from build123d import *

# Parameters (mm, degrees)
SKETCH1_R               = 4.4
BOSS_EXTRUDE1_DEPTH     = 10
SKETCH1_2_R             = 4.4
BOSS_EXTRUDE2_DEPTH     = 2
SKETCH3_W               = 30
SKETCH3_H               = 12
BOSS_EXTRUDE4_DEPTH     = 7.2
CUT_EXTRUDE2_START      = -12.2
SKETCH2_R               = 1.65
CUT_EXTRUDE2_DEPTH      = 8
SKETCH5_W               = 30
SKETCH5_H               = 3
CUT_EXTRUDE3_DEPTH      = 23.756098084
CUT_EXTRUDE3_DEPTH_BACK = 2
SKETCH6_W               = 14
SKETCH6_H               = 3
CUT_EXTRUDE4_DEPTH      = 23.756098084
CUT_EXTRUDE4_DEPTH_BACK = 23.756098084


with BuildPart() as part:
    # Sketch1 → Boss-Extrude1 (new body)
    with BuildSketch(Plane.XY):
        with BuildLine():
            Line((-15, -5), (15, -5))
            ThreePointArc((15, -5), (10.104984149, -1.836764635), (6.785093744, 2.953388374))
            ThreePointArc((6.785093744, 2.953388374), (0, 7.4), (-6.785093744, 2.953388374))
            ThreePointArc((-6.785093744, 2.953388374), (-10.104984149, -1.836764635), (-15, -5))
        make_face()
        Circle(SKETCH1_R, mode=Mode.SUBTRACT)
    extrude(amount=BOSS_EXTRUDE1_DEPTH)

    # Sketch1<2> → Boss-Extrude2 (add)
    with BuildSketch(Plane.XY):
        with BuildLine():
            ThreePointArc((-6.785093744, 2.953388374), (0, 7.4), (6.785093744, 2.953388374))
            ThreePointArc((6.785093744, 2.953388374), (10.104984149, -1.836764635), (15, -5))
            Line((15, -5), (-15, -5))
            ThreePointArc((-15, -5), (-10.104984149, -1.836764635), (-6.785093744, 2.953388374))
        make_face()
        Circle(SKETCH1_2_R, mode=Mode.SUBTRACT)
        Circle(SKETCH1_2_R)
    extrude(amount=-BOSS_EXTRUDE2_DEPTH)

    # Sketch3 → Boss-Extrude4 (add)
    with BuildSketch(Plane.XZ.offset(5)):
        with Locations((0, 4)):
            Rectangle(SKETCH3_W, SKETCH3_H)
    extrude(amount=BOSS_EXTRUDE4_DEPTH)

    # Sketch2 → Cut-Extrude2 (cut)
    with BuildSketch(Plane(origin=(0, 0, 0), x_dir=(1, 0, 0), z_dir=(0, 1, 0)).offset(CUT_EXTRUDE2_START)):
        with Locations(Location((-11.5, -4, 0), (0, 0, 90))):
            Circle(SKETCH2_R)
        with Locations(Location((11.5, -4, 0), (0, 0, 90))):
            Circle(SKETCH2_R)
    extrude(amount=CUT_EXTRUDE2_DEPTH, mode=Mode.SUBTRACT)

    # Sketch5 → Cut-Extrude3 (cut, two sides)
    with BuildSketch(Plane(origin=(0, 0, -2), x_dir=(-1, 0, 0), z_dir=(0, 0, -1))) as cut_extrude3_sk:
        with Locations((0, -10.7)):
            Rectangle(SKETCH5_W, SKETCH5_H)
    extrude(amount=CUT_EXTRUDE3_DEPTH, mode=Mode.SUBTRACT)
    extrude(cut_extrude3_sk.sketch, amount=-CUT_EXTRUDE3_DEPTH_BACK, mode=Mode.SUBTRACT)

    # Sketch6 → Cut-Extrude4 (cut, two sides)
    with BuildSketch(Plane.XY.offset(10)) as cut_extrude4_sk:
        with Locations((0, -10.7)):
            Rectangle(SKETCH6_W, SKETCH6_H)
    extrude(amount=CUT_EXTRUDE4_DEPTH, mode=Mode.SUBTRACT)
    extrude(cut_extrude4_sk.sketch, amount=-CUT_EXTRUDE4_DEPTH_BACK, mode=Mode.SUBTRACT)


solid = part.part
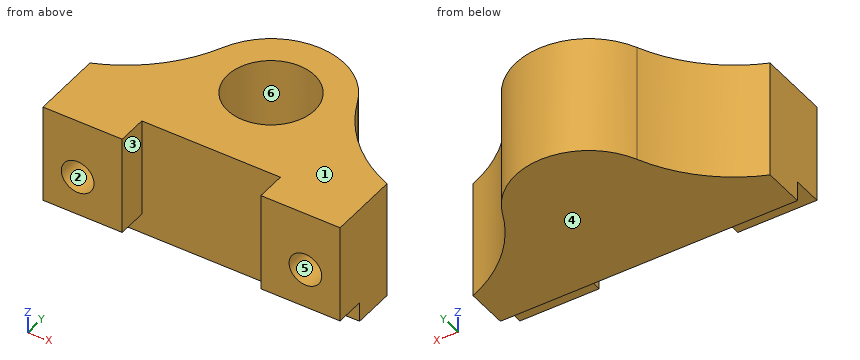
Here's how the part is built. I have some questions about the finished solid (model axes, mm). Face numbers are marked on the shaded views. A direction names the side the tool comes from. Coordinates: 2 decimals unless noted, no trailing zeros. Loops run counter-clockwise (first coordinate to the right, second up) from the corner with the lowest first, then second, coordinate; pieces in that order, holes last. Notation, with made-up numbers: (81.25, -12.5) -> (87.25, -12.5) arc R28 ccw to (87.25, 13.5) -> close; hole circle Ø8 at (27.25, 71.25). An arc over 180 degrees is marked (long way). Use one line per item in the form item = value. Start each with the question number.
(1) If we section it at A-A (y = -10): Please give me the cut outline in (x, z), then the cut area to 3 significant figures.
(2) We'd pull the mould along Z, two halves only. Please class the marked faces 4, 5 and 6: pulls with the +Z half, pulls with the -Z half, needs draft (parallel to the pull), parting line crosses it, or undercut.
(3) If we section it at D-D (x = 0): Please give me the cut outline in (y, z), then the cut area to 3 significant figures.
(4) Will these pins go through, and if not, where does the flat tip stop? pin 1 (3 mm diameter, centred on x = 8, z = 4.5, fed in from +Y); pin 2 (0.9 mm diameter, centred on x = 12.5, y = -10.5, fed in from -Z); pin 3 (2 mm diameter, centred on y = 3, z = 8.5, fed in from +X).
(5) If we section it at C-C (z = -1): Please give me the cut outline in (x, y), then the cut area to 3 significant figures.
(6) If we section it at B-B (z = 1): Please give me the cut outline in (x, y), then the cut area to 3 significant figures.
(7) On a 3-axis mill with a long thin cutter (end or side, diameter ignored), from which of +Z, -Z, +X, -X, +Y, -Y can I reach the whole of each face in a straight line? I mean the marked faces 1, 2 and 3. Say none if no direction works.
(8) Please list where these lines run through material, in increasing order: line 1 along X through (y, z) = (-8.75, 4); line 2 along Z through (x, y) = (11.5, -6); line 3 along Z through (x, y) = (-11.5, -9.75).
Verdict:
q1.outline = (-15, 0) -> (-7, 0) -> (-7, 10) -> (-15, 10) -> close; (7, 0) -> (15, 0) -> (15, 10) -> (7, 10) -> close; hole circle Ø3.3 at (-11.5, 4); hole circle Ø3.3 at (11.5, 4)
q1.area = 143 mm²
q2.face_4 = pulls with the -Z half
q2.face_5 = undercut
q2.face_6 = needs draft
q3.outline = (-9.2, -2) -> (7.4, -2) -> (7.4, 10) -> (4.4, 10) -> (4.4, 0) -> (-4.4, 0) -> (-4.4, 10) -> (-9.2, 10) -> close
q3.area = 111 mm²
q4.pin_1 = 3.54
q4.pin_2 = 0
q4.pin_3 = 7.24
q5.outline = (-15, -9.2) -> (15, -9.2) -> (15, -5) arc R15 cw to (6.79, 2.95) arc R7.4 ccw to (-6.79, 2.95) arc R15 cw to (-15, -5) -> close
q5.area = 325 mm²
q6.outline = (-15, -12.2) -> (-7, -12.2) -> (-7, -9.2) -> (7, -9.2) -> (7, -12.2) -> (15, -12.2) -> (15, -5) arc R15 cw to (6.79, 2.95) arc R7.4 ccw to (-6.79, 2.95) arc R15 cw to (-15, -5) -> close; hole circle Ø8.8 at (0, 0)
q6.area = 313 mm²
q7.face_1 = +Z, +X, -X, +Y, -Y
q7.face_2 = -Y
q7.face_3 = +Z, -Z, -Y
q8.line_1 = -15 to -13.15, -9.85 to 9.85, 13.15 to 15
q8.line_2 = -2 to 2.35, 5.65 to 10
q8.line_3 = 0 to 2.35, 5.65 to 10
